from build123d import *

# Parameters (mm, degrees)
F1_DEPTH = 25.4


with BuildPart() as f1:
    # F0 (on Front) → F1 (new body)
    with BuildSketch(Plane.XZ):
        with BuildLine():
            Line((44.391164, -51.888976), (80.822532, 80.6549))
            ThreePointArc((80.822532, 80.6549), (0, 186.69), (-80.822532, 80.6549))
            Line((-80.822532, 80.6549), (-44.391164, -51.888976))
            ThreePointArc((-44.391164, -51.888976), (0, -85.725), (44.391164, -51.888976))
        make_face()
        with BuildLine():
            Line((44.359193, 31.75), (46.0375, 31.75))
            Line((46.0375, 31.75), (46.0375, -31.75))
            Line((46.0375, -31.75), (45.348071, -31.75))
            ThreePointArc((45.348071, -31.75), (0, 6.35), (-45.348071, -31.75))
            Line((-45.348071, -31.75), (-46.0375, -31.75))
            Line((-46.0375, -31.75), (-46.0375, 31.75))
            Line((-46.0375, 31.75), (-44.359193, 31.75))
            ThreePointArc((-44.359193, 31.75), (0, 19.05), (44.359193, 31.75))
        make_face(mode=Mode.SUBTRACT)
    extrude(amount=F1_DEPTH)


solid = f1.part
The model under review builds one solid part; all positions refer to its coordinate system, in mm. A direction names the side the tool comes from. Round coordinates to 2 decimals unless told otherwise and drop trailing zeros. Order: outer loops, then holes, each group sorted by start corner. A loop starts at its lowest first (then second) coordinate and runs counter-clockwise, first axis right, second up. Notation, with made-up numbers: (80, 26) -> (139, 26) arc R7 cw to (139, 38) -> close; hole circle Ø2 at (60, -22.5). An arc over 180 degrees is marked (long way). Write item = value, one per line. Start each with the question number.
Item 1: Consider section C-C on x = -29.5. Write out the cut boundary in (y, z), plus the area to 3 significant figures.
Item 2: For faces 4 (the face through (-46.038, -13, 0)), 5 (the face through (-0.839, -12.522, -85.717)), list the 3-axis set-ups (+Z, -Z, +X, -X, +Y, -Y) from which the entire face can be reached by the end or side of a thin tool; tool diameter is ignored.
Item 3: For line 1 along X through (y, z) = (-5.25, -21); line 2 along Z through (x, y) = (27, -19); line 3 along Z through (x, y) = (25.5, -1.5), list the stretches that pass through material, from the lowest coordinate up.
Item 4: Mouldability with a two-part tool opening along Z and no side actions: class faces 1 (the face through (-1, -25.4, 83)), 2 (the face through (0.9, -12.52, 6.34)), 3 (the face through (62.352, -12.522, 13.455)) as released by +Z, released by -Z, zero draft, split by the parting line, or undercut.
Item 5: Consider section D-D on z = -54.5. Write out the cut boundary in (x, y).
Item 6: Consider section B-B on x = 0. Write out the cut boundary in (y, z) (3 decimals).
Item 7: Clearance check with flat-ended pins moving along their axes: pin 1 Ø12.5 at (y, z) = (-14.5, -0.5) entering from +X; pin 2 Ø3 at (y, z) = (-18, 62.5) entering from +X; pin 3 Ø3 at (x, y) = (-37.5, -3.5) entering from -Z. State where each tip first meets the part, or that it passes through.
Conclusion:
q1.outline = (-25.4, -75.03) -> (0, -75.03) -> (0, -4.34) -> (-25.4, -4.34) -> close; (-25.4, 24.41) -> (0, 24.41) -> (0, 181.33) -> (-25.4, 181.33) -> close
q1.area = 5,780 mm2
q2.face_4 = +Y, -Y
q2.face_5 = -Z, +Y, -Y
q3.line_1 = -52.88 to -46.04, -42.07 to 42.07, 46.04 to 52.88
q3.line_2 = -76.98 to -2.4, 23.52 to 182.22
q3.line_3 = -78.02 to -1.36, 23.02 to 182.72
q4.face_1 = zero draft
q4.face_2 = undercut
q4.face_3 = released by -Z
q5.outline = (-43.59, -25.4) -> (43.59, -25.4) -> (43.59, 0) -> (-43.59, 0) -> close
q6.outline = (-25.4, -85.725) -> (0, -85.725) -> (0, 6.35) -> (-25.4, 6.35) -> close; (-25.4, 19.05) -> (0, 19.05) -> (0, 186.69) -> (-25.4, 186.69) -> close
q7.pin_1 = 60.23
q7.pin_2 = 76.24
q7.pin_3 = -68.38
